Design review of the part built by this model. Coordinates are the model's own, in mm. Face numbers are marked on the shaded views. A direction names the side the tool comes from. Round coordinates to 2 decimals unless told otherwise and drop trailing zeros. Order: outer loops, then holes, each group sorted by start corner. A loop starts at its lowest first (then second) coordinate and runs counter-clockwise, first axis right, second up. Notation, with made-up numbers: M 16,52.25 L 65,52.25 A25 ccw 65,78.25 Z; hole C 68,22.25 d6. An arc over 180 degrees is marked long. Use a Markdown table: item, result. Add a question column.
(1) Take a section at C-C (x = -1.5). Write out the cut boundary in (y, z).
(2) The part is to be moulded in two halves that separate along X. For the marked faces 5, 6 and 7, say which applies: released by +X, released by -X, zero draft, split by the parting line, or undercut.
(3) Machinability: for the marked faces 1, 2, 3 and 4, which of the approach directions +Z, -Z, +X, -X, +Y, -Y give a long, thin tool a straight path to every point of the face, cutting with its end or side? Answer none if there is none.
(4) Take a section at D-D (y = 8.5). Write out the cut boundary in (x, z), then the cut area to 3 significant figures.
(5) Take a section at B-B (z = 4). Write out the cut boundary in (x, y), then the cut area to 3 significant figures.
(6) To check wall thickness, follow probe 1 along Y at (x, z) = (0, 5.5); probe 2 along X at (y, z) = (0.75, 1); probe 3 along X at (y, z) = (2.75, 6.25). State the ranges of each line that lie inside material, in increasing order. Write a range as from..to.
(7) For pin 1 (9.5 mm diameter, centred on x = 0, y = 0, fed in from -Z); pin 2 (5 mm diameter, centred on y = -3.5, z = 1.5, fed in from +X); pin 3 (2.5 mm diameter, centred on y = 9, z = 5, fed in from +X); pin 4 (5 mm diameter, centred on y = -3, z = 3.5, fed in from +X), all flat-tipped, find the tip position at first contact; note any pin that passes through.
(8) Take a section at A-A (y = 0). Write out the cut boundary in (x, z), then the cut area to 3 significant figures.
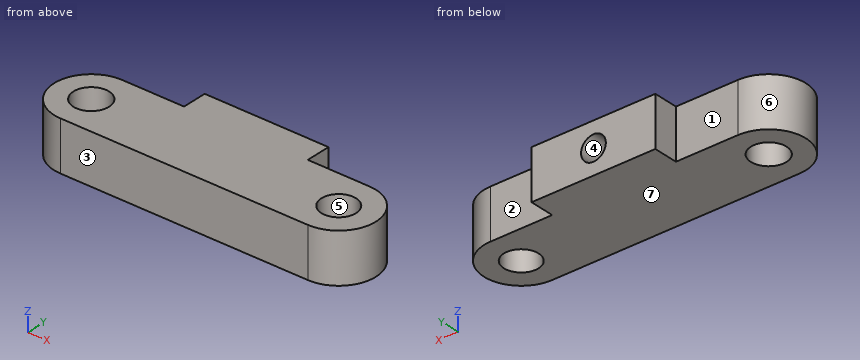
Autodesk Inventor part; units mm, degrees
ref_plane "YZ Plane" through (0, 0, 0) normal (1, 0, 0) x (0, 1, 0)
ref_plane "XZ Plane" through (0, 0, 0) normal (0, 1, 0) x (-1, 0, 0)
ref_plane "XY Plane" through (0, 0, 0) normal (0, 0, 1) x (1, 0, 0)
sketch "Sketch1" plane through (0, 0, 0) normal (0, 0, 1) x (1, 0, 0)
  circle A0 centre (0, 0) radius 3.6
  circle A1 centre (0, 0) radius 7.5 construction
  arc A2 (0, 7.5) -> (0, -7.5) centre (0, 0) ccw
  line L0 (0, 7.5) -> (50, 7.5)
  line L1 (0, -7.5) -> (50, -7.5)
  circle A3 centre (50, 0) radius 7.5 construction
  arc A4 (50, -7.5) -> (50, 7.5) centre (50, 0) ccw
  circle A5 centre (50, 0) radius 3.5
  point P0 (42.6287, 1.3837)
  point P1 (42.5553, -0.9092)
  dimension "d0" = 7.2
  dimension "d1" = 15
  dimension "d2" = 50
  dimension "d3" = 15
  dimension "d4" = 7
extrude "Extrusion1" add sketch "Sketch1" along normal blind 10
sketch "Sketch4" plane through (0, 0, 10) normal (0, 0, 1) x (1, 0, 0)
  line L0 (50, 7.5) -> (0, 7.5)
  line L1 (12.5, 7.5) -> (37.5, 7.5)
  line L2 (37.5, 7.5) -> (37.5, 12.5)
  line L3 (37.5, 12.5) -> (12.5, 12.5)
  line L4 (12.5, 12.5) -> (12.5, 7.5)
  point P0 (0, 0)
  point P1 (25, 7.5)
  dimension "d10" = 25
  dimension "d11" = 5
extrude "Extrusion3" add sketch "Sketch4" against normal blind 10
sketch "Sketch5" plane through (12.5, 12.5, 10) normal (0, 1, 0) x (1, 0, 0)
  line L0 (25, 0) -> (0, 0)
  line L1 (25, 0) -> (25, 10)
  line L2 (0, 10) -> (25, 10)
  line L3 (0, 0) -> (0, 10)
  circle A0 centre (12.5, 5) radius 2.5
  line L4 (0, 0) -> (0, 10)
  point P0 (-12.5, 10)
  point P1 (12.5, 10)
  point P2 (0, 5)
  dimension "d14" = 5
extrude "Extrusion4" cut sketch "Sketch5" against normal blind 10 contours A0
properties part number "GA003" material "ABS Plastic"
Verdict:
| question | item | result |
|---|---|---|
| 1 | outline | M -7.35,0 L -3.27,0 L -3.27,10 L -7.35,10 Z; M 3.27,0 L 7.35,0 L 7.35,10 L 3.27,10 Z |
| 2 | face 5 | undercut |
| 2 | face 6 | released by -X |
| 2 | face 7 | zero draft |
| 3 | face 1 | +Z, -Z, -X, +Y |
| 3 | face 2 | +Z, -Z, +X, +Y |
| 3 | face 3 | +Z, -Z, +X, -X, -Y |
| 3 | face 4 | +Y |
| 4 | outline | M 12.5,0 L 37.5,0 L 37.5,10 L 12.5,10 Z; hole C 25,5 d5 |
| 4 | area | 230 mm^2 |
| 5 | outline | M 0,-7.5 L 50,-7.5 A7.5 ccw 50,7.5 L 37.5,7.5 L 37.5,12.5 L 27.29,12.5 L 27.29,2.5 L 22.71,2.5 L 22.71,12.5 L 12.5,12.5 L 12.5,7.5 L 0,7.5 A7.5 ccw Z; hole C 0,0 d7.2; hole C 50,0 d7 |
| 5 | area | 927 mm^2 |
| 6 | probe 1 | y = -7.5..-3.6, 3.6..7.5 |
| 6 | probe 2 | x = -7.46..-3.52, 3.52..46.58, 53.42..57.46 |
| 6 | probe 3 | x = -6.98..-2.32, 2.32..22.83, 27.17..47.83, 52.17..56.98 |
| 7 | pin 1 | stops at z = 0 |
| 7 | pin 2 | stops at x = 57.43 |
| 7 | pin 3 | stops at x = 37.5 |
| 7 | pin 4 | stops at x = 57.48 |
| 8 | outline | M -7.5,0 L -3.6,0 L -3.6,10 L -7.5,10 Z; M 3.6,0 L 46.5,0 L 46.5,10 L 3.6,10 Z; M 53.5,0 L 57.5,0 L 57.5,10 L 53.5,10 Z |
| 8 | area | 508 mm^2 |
